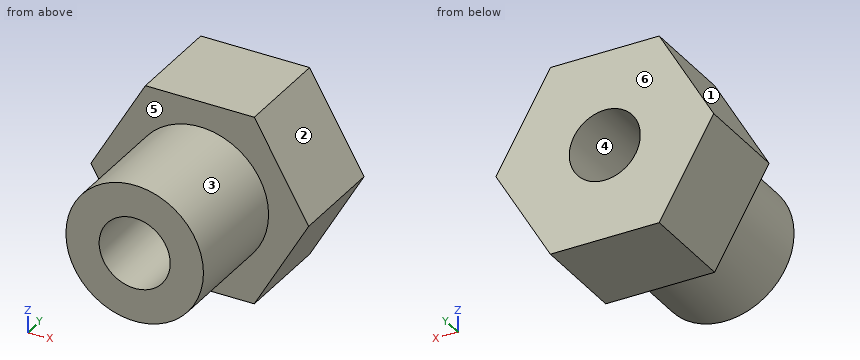
Autodesk Inventor part; units mm, degrees
ref_plane "YZ Plane" through (0, 0, 0) normal (1, 0, 0) x (0, 1, 0)
ref_plane "XZ Plane" through (0, 0, 0) normal (0, 1, 0) x (-1, 0, 0)
ref_plane "XY Plane" through (0, 0, 0) normal (0, 0, 1) x (1, 0, 0)
sketch "Sketch1" plane through (0, 0, 0) normal (0, 1, 0) x (-1, 0, 0)
  line L0 (-9.5, 0) -> (-4.75, 8.2272)
  line L1 (-4.75, 8.2272) -> (4.75, 8.2272)
  line L2 (4.75, 8.2272) -> (9.5, 0)
  line L3 (9.5, 0) -> (4.75, -8.2272)
  line L4 (4.75, -8.2272) -> (-4.75, -8.2272)
  line L5 (-4.75, -8.2272) -> (-9.5, 0)
  point P0 (0, 0)
  point P1 (0, 0)
  dimension "d2" = 9.5
extrude "Extrusion1" add sketch "Sketch1" along normal blind 8.5
sketch "Sketch2" plane through (0, 0, 0) normal (0, -1, 0) x (1, 0, 0)
  circle A0 centre (0, 0) radius 6
  circle A1 centre (0, 0) radius 3.1
  dimension "d5" = 12
  dimension "d6" = 6.2
extrude "Extrusion2" add sketch "Sketch2" along normal blind 10
sketch "Sketch3" plane through (0, 0, 0) normal (0, -1, 0) x (1, 0, 0)
  circle A0 centre (0, 0) radius 3.1
extrude "Extrusion3" cut sketch "Sketch3" against normal through all
thread "Thread1"
properties part number "Premistoppa"
For this review, take the finished solid that the model builds, in its own axes (mm). Face numbers are marked on the shaded views. A direction names the side the tool comes from. Round coordinates to 2 decimals unless told otherwise and drop trailing zeros. Order: outer loops, then holes, each group sorted by start corner. A loop starts at its lowest first (then second) coordinate and runs counter-clockwise, first axis right, second up. Notation, with made-up numbers: M 53,51 L 83,51 A35 ccw 83,83 Z; hole C 88,48 d10. An arc over 180 degrees is marked long. Use a Markdown table: item, result. Add a question column.
Item 1: Insertion check: pin 1 (4 mm diameter, centred on x = -5, y = 2.5, fed in from +Z); pin 2 (6 mm diameter, centred on y = -6.5, z = 4, fed in from -X); pin 3 (5 mm diameter, centred on y = 4, z = 2, fed in from +X); pin 4 (6 mm diameter, centred on y = 2.5, z = 4.5, fed in from -X). Each pin has a flat end and moves straight along its axis. Give the tip position at first contact, or say it passes through.
Item 2: Add section D-D, the plane z = -4. Give the boundary of the cut face in (x, y), then the cut area to 3 significant figures.
Item 3: Add section B-B, the plane x = 0. Give the boundary of the cut face in (y, z), then the cut area to 3 significant figures.
Item 4: Add section A-A, the plane y = 7.25. Give the boundary of the cut face in (x, z).
Item 5: To check wall thickness, follow line 1 along Z through (x, y) = (0, 4.25); line 2 along Y through (x, z) = (-1.25, 7.25); line 3 along X through (y, z) = (4.75, 2.5). State the ranges of each line that lie inside material, in increasing order.
Item 6: Mouldability with a two-part tool opening along X and no side actions: class the marked faces 1, 2, 3 and 4 as released by +X, released by -X, zero draft, split by the parting line, or undercut.
Item 7: Add section C-C, the plane z = -2. Give the boundary of the cut face in (x, y).
Item 8: Tool access review of the marked faces 5 and 6: name each direction out of +Z, -Z, +X, -X, +Y, -Y from which nothing blocks a thin tool from reaching the whole face with its end or side.
Geometry results:
| question | item | result |
|---|---|---|
| 1 | pin 1 | stops at z = 8.23 |
| 1 | pin 2 | stops at x = -5.92 |
| 1 | pin 3 | stops at x = 9.5 |
| 1 | pin 4 | stops at x = -8.63 |
| 2 | outline | M -7.19,0 L -4.47,0 L -4.47,-10 L 4.47,-10 L 4.47,0 L 7.19,0 L 7.19,8.5 L -7.19,8.5 Z |
| 2 | area | 212 mm² |
| 3 | outline | M -10,-6 L 0,-6 L 0,-8.23 L 8.5,-8.23 L 8.5,-3.1 L -10,-3.1 Z; M -10,3.1 L 8.5,3.1 L 8.5,8.23 L 0,8.23 L 0,6 L -10,6 Z |
| 3 | area | 145 mm² |
| 4 | outline | M -9.5,0 L -4.75,-8.23 L 4.75,-8.23 L 9.5,0 L 4.75,8.23 L -4.75,8.23 Z; hole C 0,0 d6.2 |
| 5 | line 1 | z = -8.23 to -3.1, 3.1 to 8.23 |
| 5 | line 2 | y = 0 to 8.5 |
| 5 | line 3 | x = -8.06 to -1.83, 1.83 to 8.06 |
| 6 | face 1 | released by -X |
| 6 | face 2 | released by +X |
| 6 | face 3 | split by the parting line |
| 6 | face 4 | undercut |
| 7 | outline | M -8.35,0 L -5.66,0 L -5.66,-10 L -2.37,-10 L -2.37,8.5 L -8.35,8.5 Z; M 2.37,-10 L 5.66,-10 L 5.66,0 L 8.35,0 L 8.35,8.5 L 2.37,8.5 Z |
| 8 | face 5 | -Y |
| 8 | face 6 | +Z, -Z, +X, -X, +Y |
